Model file for the job. Use its own axes, mm. Face numbers are marked on the shaded views. A direction names the side the tool comes from. Give positions to 0.01 mm unless a question says otherwise; leave off trailing zeros. Order: outer loops, then holes, each group sorted by start corner. A loop starts at its lowest first (then second) coordinate and runs counter-clockwise, first axis right, second up. Notation, with made-up numbers: (6, 71.25) - (32, 71.25) arc R19 ccw to (32, 99.25) - close; hole circle Ø4 at (86.25, 56). An arc over 180 degrees is marked (long way). Use CSV: the item, a comma, the result in double quotes. Start each with the question number.
(1) Pull direction X, two halves, no side cores. Call the marked faces 1, 2 and 3: +X half, -X half, draft (parallel to the pull), parting line (faces both ways), or undercut.
(2) Tool access for the marked faces 4, 5 and 6: list every direction of +Z, -Z, +X, -X, +Y, -Y with a clear straight run to the whole face (end or side of a thin tool).
(3) Band-saw the part on A-A, the plane y = -15. Give the cut face in (x, z).
(4) Probe L1, parallel to X at y = -40, z = 27; L2, parallel to Y at x = -17.5, z = 3.1. List the from-to ranges inside material, lowest first.
(5) Band-saw the part on D-D, the plane x = -13. Give the cut face in (y, z), then the cut area to 3 significant figures.
(6) Band-saw the part on B-B, the plane x = -1.5. Give the cut face in (y, z), then the cut area to 3 significant figures.
(7) Drop flat-ended pins along their axis: pin 1 Ø5 at (x, z) = (0, 0) entering from -Y; pin 2 Ø2 at (x, z) = (0, 22.5) entering from +Y; pin 3 Ø3 at (x, z) = (11.5, 1) entering from -Y. Give the stop position or say it passes through.
(8) Band-saw the part on C-C, the plane y = -9. Give the cut face in (x, z).
from build123d import *

# Parameters (mm, degrees)
SKETCH1_R           = 4
SKETCH1_R_2         = 3
SKETCH3_R           = 2
BOSS_EXTRUDE1_DEPTH = 2
FILLET1_R           = 8


with BuildPart() as part:
    # Sweep1: sweep along a path in Sketch2
    with BuildLine(Plane(origin=(0, 0, 0), x_dir=(0, 0, -1), z_dir=(1, 0, 0))) as sweep1_path:
        Line((0, 0), (0, -30))
        Line((0, -30), (-28.190778624, -40.2606043))
    # Sketch1 → Sweep1 (sweep)
    with BuildSketch(Plane(origin=(0, 0, 0), x_dir=(1, 0, 0), z_dir=(0, 1, 0))):
        Circle(SKETCH1_R)
        Circle(SKETCH1_R_2, mode=Mode.SUBTRACT)
    sweep(path=sweep1_path.line, transition=Transition.RIGHT)

    # Sketch3 → Boss-Extrude1 (add)
    with BuildSketch(Plane.XY.offset(4)):
        with BuildLine():
            Line((17.5, -20), (-17.5, -20))
            ThreePointArc((-17.5, -20), (-22.5, -15), (-17.5, -10))
            Line((-17.5, -10), (17.5, -10))
            ThreePointArc((17.5, -10), (22.5, -15), (17.5, -20))
        make_face()
        with Locations((17.5, -15)):
            Circle(SKETCH3_R, mode=Mode.SUBTRACT)
        with Locations((-17.5, -15)):
            Circle(SKETCH3_R, mode=Mode.SUBTRACT)
    extrude(amount=-BOSS_EXTRUDE1_DEPTH)

    # Fillet1
    # the kernel refuses this fillet: 8 mm, written as the material it adds along each edge
    with BuildSketch(Plane(origin=(-3.464101615, -10, 2), x_dir=(0, 0, -1), z_dir=(0, -1, 0))) as fillet1_piece_1:
        with BuildLine():
            CenterArc((8, -6.92820323), FILLET1_R, 120, 60)
            Line((0, -6.92820323), (0, 0))
            ThreePointArc((0, 0), (2, -0.535898385), (4, 0))
        make_face()
    extrude(amount=10)
    with BuildSketch(Plane(origin=(3.464101615, -10, 2), x_dir=(0, 0, -1), z_dir=(0, -1, 0))) as fillet1_piece_2:
        with BuildLine():
            CenterArc((8, 6.92820323), FILLET1_R, 180, 60)
            Line((0, 6.92820323), (0, 0))
            ThreePointArc((0, 0), (2, 0.535898385), (4, 0))
        make_face()
    extrude(amount=10)


solid = part.part
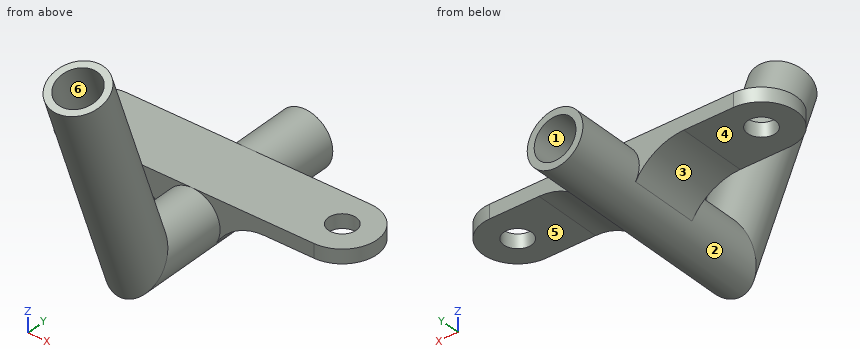
Answer block:
1,face 1,"undercut"
1,face 2,"parting line"
1,face 3,"-X half"
2,face 4,"-Z, -X, +Y, -Y"
2,face 5,"-Z, +X, +Y, -Y"
2,face 6,"none"
3,outline,"(-22.5, 2) - (-19.5, 2) - (-19.5, 4) - (-22.5, 4) - close; (-15.5, 2) - (-10.39, 2) arc R8 cw to (-3.46, -2) arc R4 ccw to (3.46, -2) arc R8 cw to (10.39, 2) - (15.5, 2) - (15.5, 4) - (-15.5, 4) - close; (19.5, 2) - (22.5, 2) - (22.5, 4) - (19.5, 4) - close; hole (-2.24, 2) arc R3 ccw (long way) to (2.24, 2) - close"
4,L1,"x = -4 to -3, 3 to 4"
4,L2,"y = -20 to -17, -13 to -10"
5,outline,"(-20, 2) - (-10, 2) - (-10, 4) - (-20, 4) - close"
5,area,"20.0 mm2"
6,outline,"(-43.75, 26.92) - (-32.6, -3.71) - (0, -3.71) - (0, -2.6) - (-31.82, -2.6) - (-42.7, 27.3) - close; (-37.82, 29.08) - (-28.18, 2.6) - (-20, 2.6) - (-20, 2) - (-10, 2) - (-10, 2.6) - (0, 2.6) - (0, 3.71) - (-10, 3.71) - (-10, 4) - (-20, 4) - (-20, 3.71) - (-27.4, 3.71) - (-36.78, 29.46) - close"
6,area,"142 mm2"
7,pin 1,"stops at y = -35.17"
7,pin 2,"stops at y = -33.57"
7,pin 3,"stops at y = -20"
8,outline,"circle Ø8 at (0, 0); hole circle Ø6 at (0, 0)"
